Geometry: see drawing. Coordinates: mm, zero at the bounding-box minimum. Give positions to 0.01 mm unless a question says otherwise; leave off trailing zeros. Write each loop counter-clockwise with the first axis right and the second up, starting at its lowest first coordinate (ties: lowest second). Pieces come first, ordered by that corner, then holes. Notation, with made-up numbers: (69, 29) - (83, 29) arc R17 ccw to (83, 43) - close; hole circle Ø3 at (68.5, 61.5). An arc over 180 degrees is marked (long way). Use a Markdown table: item, result. Add a question column.
1. Material intervals for probe 1 along Y at (x, z) = (152.75, 1.55); probe 2 along X at (y, z) = (70.75, 0.85); probe 3 along X at (y, z) = (22, 0.3), sorted ascending.
2. Section query B-B, the plane y = 42.75. Return loops of the section in (x, z).
3. Section query A-A, the plane x = 110.75. Return loops of the section in (y, z), plus the area to 3 significant figures.
4. Section query C-C, the plane z = 0.5. Return loops of the section in (x, y).
5. Pin query (flat end, axial travel): pin 1 (1.5 mm diameter, centred on x = 4, z = 2, fed in from +Y). Return the tip coordinate at first contact, or that it passes through.
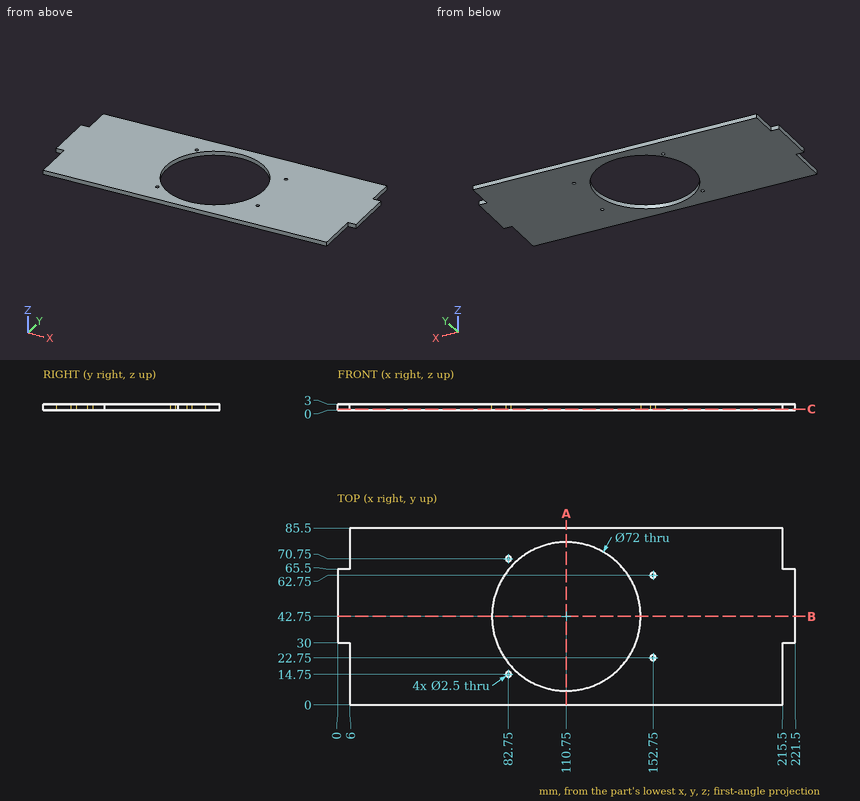
Result sheet:
| question | item | result |
|---|---|---|
| 1 | probe 1 | y = 0 to 21.5, 24 to 61.5, 64 to 85.5 |
| 1 | probe 2 | x = 6 to 81.5, 84 to 88.12, 133.38 to 215.5 |
| 1 | probe 3 | x = 6 to 81.33, 140.17 to 151.75, 153.75 to 215.5 |
| 2 | outline | (0, 0) - (74.75, 0) - (74.75, 3) - (0, 3) - close; (146.75, 0) - (221.5, 0) - (221.5, 3) - (146.75, 3) - close |
| 3 | outline | (0, 0) - (6.75, 0) - (6.75, 3) - (0, 3) - close; (78.75, 0) - (85.5, 0) - (85.5, 3) - (78.75, 3) - close |
| 3 | area | 40.5 mm² |
| 4 | outline | (0, 30) - (6, 30) - (6, 0) - (215.5, 0) - (215.5, 30) - (221.5, 30) - (221.5, 65.5) - (215.5, 65.5) - (215.5, 85.5) - (6, 85.5) - (6, 65.5) - (0, 65.5) - close; hole circle Ø72 at (110.75, 42.75); hole circle Ø2.5 at (82.75, 14.75); hole circle Ø2.5 at (82.75, 70.75); hole circle Ø2.5 at (152.75, 22.75); hole circle Ø2.5 at (152.75, 62.75) |
| 5 | pin 1 | stops at y = 65.5 |
